from build123d import *

# Parameters (mm, degrees)
SKETCH1_W            = 54.33
SKETCH1_H            = 39.33
BOSS_EXTRUDE1_DEPTH  = 1
SKETCH2_W            = 6.7
SKETCH2_H            = 1.65
BOSS_EXTRUDE2_DEPTH  = 1
SKETCH3_W            = 20.51
SKETCH3_H            = 4.6
BOSS_EXTRUDE3_DEPTH  = 1
SKETCH5_W            = 50.087359313
SKETCH5_H            = 35.087359313
CUT_EXTRUDE1_DEPTH   = 11
SKETCH6_W            = 18.5
SKETCH6_H            = 7.9
BOSS_EXTRUDE5_DEPTH  = 1
SKETCH7_W            = 20.51
SKETCH7_H            = 1
CUT_EXTRUDE3_DEPTH   = 4.6
SKETCH10_W           = 8
SKETCH10_H           = 1
SKETCH10_W_2         = 5.6
BOSS_EXTRUDE8_DEPTH  = 54.33
SKETCH11_W           = 8.7
SKETCH11_H           = 1
BOSS_EXTRUDE9_DEPTH  = 39.33
SKETCH12_W           = 20.5
SKETCH12_H           = 1
BOSS_EXTRUDE10_DEPTH = 6.25
SKETCH13_W           = 2
SKETCH13_H           = 25.73
BOSS_EXTRUDE14_DEPTH = 2.6
SKETCH16_W           = 25.73
SKETCH16_H           = 1
BOSS_EXTRUDE15_DEPTH = 4
SKETCH17_W           = 25.73
SKETCH17_H           = 1
BOSS_EXTRUDE16_DEPTH = 4


with BuildPart() as part:
    # Sketch1 → Boss-Extrude1 (new body)
    with BuildSketch(Plane(origin=(0, 0, 0), x_dir=(1, 0, 0), z_dir=(0, 1, 0))):
        with Locations((-6.631882129, 3.775979087)):
            Rectangle(SKETCH1_W, SKETCH1_H)
    extrude(amount=BOSS_EXTRUDE1_DEPTH)

    # Sketch2 → Boss-Extrude2 (add)
    with BuildSketch(Plane(origin=(20.533117871, 0, 0), x_dir=(0, 0, -1), z_dir=(1, 0, 0))):
        with Locations((-6.719020913, -0.825)):
            Rectangle(SKETCH2_W, SKETCH2_H)
    extrude(amount=-BOSS_EXTRUDE2_DEPTH)

    # Sketch3 → Boss-Extrude3 (add)
    with BuildSketch(Plane.XY.offset(15.889020913)):
        with Locations((-6.431882129, -2.3)):
            Rectangle(SKETCH3_W, SKETCH3_H)
    extrude(amount=-BOSS_EXTRUDE3_DEPTH)

    # Sketch5 → Cut-Extrude1 (cut)
    with BuildSketch(Plane(origin=(0, 1, 0), x_dir=(1, 0, 0), z_dir=(0, 1, 0))):
        with Locations((-6.63188213, 3.775979088)):
            Rectangle(SKETCH5_W, SKETCH5_H)
    extrude(amount=-CUT_EXTRUDE1_DEPTH, mode=Mode.SUBTRACT)

    # Sketch6 → Boss-Extrude5 (add)
    with BuildSketch(Plane(origin=(0, 0, -23.440979087), x_dir=(-1, 0, 0), z_dir=(0, 0, -1))):
        with Locations((6.426882129, -3.95)):
            Rectangle(SKETCH6_W, SKETCH6_H)
    extrude(amount=-BOSS_EXTRUDE5_DEPTH)

    # Sketch7 → Cut-Extrude3 (cut)
    with BuildSketch(Plane.XZ.offset(4.6)):
        with Locations((-6.431882129, 15.389020913)):
            Rectangle(SKETCH7_W, SKETCH7_H)
    extrude(amount=-CUT_EXTRUDE3_DEPTH, mode=Mode.SUBTRACT)

    # Sketch10 → Boss-Extrude8 (add)
    with BuildSketch(Plane.ZY.offset(33.796882129)):
        with Locations((11.889020913, 0.5)):
            Rectangle(SKETCH10_W, SKETCH10_H)
        with Locations((-20.640979087, 0.5)):
            Rectangle(SKETCH10_W_2, SKETCH10_H)
    extrude(amount=-BOSS_EXTRUDE8_DEPTH)

    # Sketch11 → Boss-Extrude9 (add)
    with BuildSketch(Plane.XY.offset(15.889020913)):
        with Locations((16.183117871, 0.5)):
            Rectangle(SKETCH11_W, SKETCH11_H)
        with Locations((-29.446882129, 0.5)):
            Rectangle(SKETCH11_W, SKETCH11_H)
    extrude(amount=-BOSS_EXTRUDE9_DEPTH)

    # Sketch12 → Boss-Extrude10 (add)
    with BuildSketch(Plane(origin=(0, 0, -23.440979087), x_dir=(-1, 0, 0), z_dir=(0, 0, -1))):
        with Locations((6.426882129, -7.4)):
            Rectangle(SKETCH12_W, SKETCH12_H)
    extrude(amount=BOSS_EXTRUDE10_DEPTH)

    # Sketch13 → Boss-Extrude14 (add)
    with BuildSketch(Plane.XZ):
        with Locations((16.833117871, -4.975979087)):
            Rectangle(SKETCH13_W, SKETCH13_H)
        with Locations((-30.096882129, -4.975979087)):
            Rectangle(SKETCH13_W, SKETCH13_H)
    extrude(amount=BOSS_EXTRUDE14_DEPTH)

    # Sketch16 → Boss-Extrude15 (add)
    with BuildSketch(Plane.ZY.offset(-15.833117871)):
        with Locations((-4.975979087, -2.1)):
            Rectangle(SKETCH16_W, SKETCH16_H)
    extrude(amount=BOSS_EXTRUDE15_DEPTH)

    # Sketch17 → Boss-Extrude16 (add)
    with BuildSketch(Plane(origin=(-29.096882129, 0, 0), x_dir=(0, 0, -1), z_dir=(1, 0, 0))):
        with Locations((4.975979087, -2.1)):
            Rectangle(SKETCH17_W, SKETCH17_H)
    extrude(amount=BOSS_EXTRUDE16_DEPTH)


solid = part.part
The listing builds one solid part. Answer for the finished solid, in the listing's coordinates (mm). A direction names the side the tool comes from. Give positions to 0.01 mm unless a question says otherwise; leave off trailing zeros. Write each loop counter-clockwise with the first axis right and the second up, starting at its lowest first coordinate (ties: lowest second). Pieces come first, ordered by that corner, then holes. Notation, with made-up numbers: (68.5, 60) - (74.5, 60) arc R22 ccw to (74.5, 92) - close; hole circle Ø8 at (-7, 11.5). An arc over 180 degrees is marked (long way). Use a Markdown table: item, result.
1. Section B-B on x = -14.5 is taken. Write down the section's boundary in (y, z).
Values follow:
| item | result |
|---|---|
| outline | (-7.9, -29.69) - (-6.9, -29.69) - (-6.9, -23.44) - (1, -23.44) - (1, -17.84) - (0, -17.84) - (0, -22.44) - (-7.9, -22.44) - close; (0, 7.89) - (1, 7.89) - (1, 15.89) - (0, 15.89) - close |
2. For a pull along X with two mould halves and no side action, classify faces 6 (the flat face through (-29, -2, -17.841)), 7 (the flat face through (-13, 0, 9)), 8 (the flat face through (-31.097, -1, -5)) as released by +X, released by -X, zero draft, split by the parting line, or undercut.
Values follow:
| item | result |
|---|---|
| face 6 | zero draft |
| face 7 | undercut |
| face 8 | released by -X |
3. Section A-A on z = -14 is taken. Write down the section's boundary in (x, y).
Values follow:
| item | result |
|---|---|
| outline | (-33.8, 0) - (-31.1, 0) - (-31.1, -2.6) - (-25.1, -2.6) - (-25.1, -1.6) - (-29.1, -1.6) - (-29.1, 0) - (-25.1, 0) - (-25.1, 1) - (-33.8, 1) - close; (11.83, -2.6) - (17.83, -2.6) - (17.83, 0) - (20.53, 0) - (20.53, 1) - (11.83, 1) - (11.83, 0) - (15.83, 0) - (15.83, -1.6) - (11.83, -1.6) - close |
4. A tool of negligible diameter and unlimited length cuts with its end or side. For faces 1 (the flat face through (15.833, -1, -5)), 2 (the flat face through (16, -2, -17.841)), 3 (the flat face through (-6, -4, -22.441)), 4 (the flat face through (17.833, -1, -5)), 5 (the flat face through (-29, -2, 7.889)), from which of +Z, -Z, +X, -X, +Y, -Y can it reach the whole face along a straight path? Write none if from no direction.
Values follow:
| item | result |
|---|---|
| face 1 | +Z, -Z |
| face 2 | -Z, +X, -X, -Y |
| face 3 | +Z, +X, -X, -Y |
| face 4 | +Z, -Z, -Y |
| face 5 | +Z, -X, -Y |
5. Each of these flat-tipped pins is pushed along its axis until it touches: P1, Ø0.8, axis at x = 20, y = -1, coming from the -Z side; P2, Ø0.8, axis at x = -27.5, y = -1.5, coming from the +Z side; P3, Ø2, axis at y = -1.5, z = -6, coming from the -X side. Where does it stop, or does it pass through?
Values follow:
| item | result |
|---|---|
| P1 | stops at z = 3.37 |
| P2 | stops at z = 7.89 |
| P3 | stops at x = -31.1 |
6. Section D-D on x = -24 is taken. Write down the section's boundary in (y, z), plus the area to 3 significant figures.
Values follow:
| item | result |
|---|---|
| outline | (0, -23.44) - (1, -23.44) - (1, -17.84) - (0, -17.84) - close; (0, 7.89) - (1, 7.89) - (1, 15.89) - (0, 15.89) - close |
| area | 13.6 mm² |
7. Find the intervals of material crossed by probe 1 along Z at (x, y) = (-21.5, 0.5); probe 2 along X at (y, z) = (-2.25, -3); probe 3 along Z at (x, y) = (-2, -6.5), in increasing order. Write a range as from..to.
Values follow:
| item | result |
|---|---|
| probe 1 | z = -23.44..-17.84, 7.89..15.89 |
| probe 2 | x = -31.1..-25.1, 11.83..17.83 |
| probe 3 | z = -23.44..-22.44 |
8. Section C-C on z = 4 is taken. Write down the section's boundary in (x, y), plus the area to 4 significant figures.
Values follow:
| item | result |
|---|---|
| outline | (-33.8, 0) - (-31.1, 0) - (-31.1, -2.6) - (-25.1, -2.6) - (-25.1, -1.6) - (-29.1, -1.6) - (-29.1, 0) - (-25.1, 0) - (-25.1, 1) - (-33.8, 1) - close; (11.83, -2.6) - (17.83, -2.6) - (17.83, 0) - (19.53, 0) - (19.53, -1.65) - (20.53, -1.65) - (20.53, 1) - (11.83, 1) - (11.83, 0) - (15.83, 0) - (15.83, -1.6) - (11.83, -1.6) - close |
| area | 37.45 mm² |
